Model file for the job. Use its own axes, mm. Face numbers are marked on the shaded views. Coordinates: 2 decimals unless noted, no trailing zeros. Order: outer loops, then holes, each group sorted by start corner. A loop starts at its lowest first (then second) coordinate and runs counter-clockwise, first axis right, second up. Notation, with made-up numbers: M 25,52 L 70,52 A20 cw 70,64 Z; hole C -7,-32.5 d4. An arc over 180 degrees is marked long. Return JSON: item names as keys, results as strings.
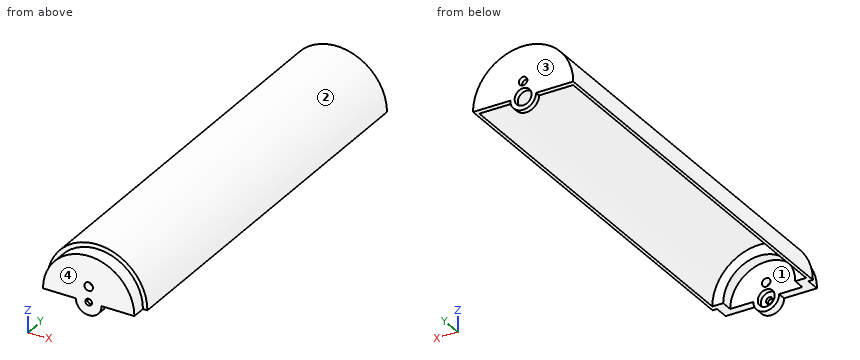
```python
from build123d import *
from build123d.topology import SkipClean

# Parameters (mm, degrees)
BOSS_EXTRUDE1_DEPTH      = 3.81
BOSS_EXTRUDE1_DEPTH_BACK = 6.35
SKETCH1_R                = 49.4538
SKETCH2_R                = 49.4538
BOSS_EXTRUDE2_DEPTH      = 381
SHELL1_T                 = -3.175
CUT_EXTRUDE1_DEPTH       = 398.363186857
BOSS_EXTRUDE3_DEPTH      = 3.81
SKETCH7_R                = 49.4538
SKETCH7_R_2              = 45.085
CUT_EXTRUDE2_DEPTH       = 6.35
BOSS_EXTRUDE4_START      = 7.62
BOSS_EXTRUDE4_DEPTH      = 7.62
SKETCH10_R               = 35.56
CUT_EXTRUDE3_DEPTH       = 6.35
SKETCH11_R               = 8.382
CUT_EXTRUDE4_DEPTH       = 5.08
SKETCH12_R               = 3.302
CUT_EXTRUDE5_DEPTH       = 402.739558289
BOSS_EXTRUDE5_DEPTH      = 5.08
SKETCH14_R               = 4.191
CUT_EXTRUDE6_DEPTH       = 405.866453376
BOSS_EXTRUDE6_DEPTH      = 5.08
SKETCH16_R               = 8.382
CUT_EXTRUDE7_DEPTH       = 405.866453376
CUT_EXTRUDE8_REACH       = 411.871
SKETCH17_R               = 4.191


with BuildPart() as part:
    # Sketch1 → Boss-Extrude1 (new, two sides: drawn at the far end of the back side and taken through both)
    with BuildSketch(Plane(origin=(0, 0, 0), x_dir=(1, 0, 0), z_dir=(0, 1, 0)).offset(-BOSS_EXTRUDE1_DEPTH_BACK)):
        with Locations(Location((0, 0, 0), (0, 0, 270))):
            Circle(SKETCH1_R)
    extrude(amount=BOSS_EXTRUDE1_DEPTH + BOSS_EXTRUDE1_DEPTH_BACK)

    # Sketch2 → Boss-Extrude2 (add)
    with BuildSketch(Plane(origin=(0, 3.81, 0), x_dir=(1, 0, 0), z_dir=(0, 1, 0))):
        with Locations(Location((0, 0, 0), (0, 0, 270))):
            Circle(SKETCH2_R)
    extrude(amount=BOSS_EXTRUDE2_DEPTH)

    # Shell1
    shell1_openings = [part.faces().sort_by_distance(p)[0] for p in [
        (0, 384.81, 0),
    ]]
    offset(amount=SHELL1_T, openings=shell1_openings, kind=Kind.INTERSECTION)

    # Sketch4 → Cut-Extrude1 (cut, through all)
    with BuildSketch(Plane.XZ.offset(6.35)):
        with BuildLine():
            Line((49.4538, 0), (12.7, 0))
            ThreePointArc((12.7, 0), (0, -12.7), (-12.7, 0))
            Line((-12.7, 0), (-49.4538, 0))
            ThreePointArc((-49.4538, 0), (0, -49.4538), (49.4538, 0))
        make_face()
    extrude(amount=-CUT_EXTRUDE1_DEPTH, mode=Mode.SUBTRACT)

    # Sketch5 → Boss-Extrude3 (add)
    with BuildSketch(Plane(origin=(0, -3.175, 0), x_dir=(1, 0, 0), z_dir=(0, 1, 0))):
        with BuildLine():
            Line((-46.2788, 0), (-12.7, 0))
            ThreePointArc((-12.7, 0), (0, 12.7), (12.7, 0))
            Line((12.7, 0), (46.2788, 0))
            ThreePointArc((46.2788, 0), (0, -46.2788), (-46.2788, 0))
        make_face()
    extrude(amount=BOSS_EXTRUDE3_DEPTH)

    # Sketch7 → Cut-Extrude2 (cut)
    with BuildSketch(Plane.XZ.offset(6.35)):
        Circle(SKETCH7_R)
        Circle(SKETCH7_R_2, mode=Mode.SUBTRACT)
    extrude(amount=-CUT_EXTRUDE2_DEPTH, mode=Mode.SUBTRACT)

    # Sketch9 → Boss-Extrude4 (add)
    with SkipClean():  # the faces are left unmerged after this step: merging them gives an invalid solid
        with BuildSketch(Plane.XZ.offset(6.35).offset(BOSS_EXTRUDE4_START)):
            with BuildLine():
                Line((45.085, 0), (12.7, 0))
                ThreePointArc((12.7, 0), (0, -12.7), (-12.7, 0))
                Line((-12.7, 0), (-45.085, 0))
                ThreePointArc((-45.085, 0), (0, 45.085), (45.085, 0))
            make_face()
        extrude(amount=-BOSS_EXTRUDE4_DEPTH)
    add(part.part.scale(1), mode=Mode.REPLACE)  # the faces are merged on a copy

    # Sketch10 → Cut-Extrude3 (cut)
    with BuildSketch(Plane(origin=(0, 0.635, 0), x_dir=(1, 0, 0), z_dir=(0, 1, 0))):
        Circle(SKETCH10_R)
    extrude(amount=-CUT_EXTRUDE3_DEPTH, mode=Mode.SUBTRACT)

    # Sketch11 → Cut-Extrude4 (cut)
    with BuildSketch(Plane(origin=(0, -5.715, 0), x_dir=(1, 0, 0), z_dir=(0, 1, 0))):
        with Locations(Location((0, 0, 0), (0, 0, 270))):
            Circle(SKETCH11_R)
    extrude(amount=-CUT_EXTRUDE4_DEPTH, mode=Mode.SUBTRACT)

    # Sketch12 → Cut-Extrude5 (cut, through all)
    with BuildSketch(Plane(origin=(0, -10.795, 0), x_dir=(1, 0, 0), z_dir=(0, 1, 0))):
        with Locations(Location((0, 0, 0), (0, 0, 270))):
            Circle(SKETCH12_R)
    extrude(amount=-CUT_EXTRUDE5_DEPTH, mode=Mode.SUBTRACT)

    # Sketch13 → Boss-Extrude5 (add)
    with SkipClean():  # the faces are left unmerged after this step: merging them gives an invalid solid
        with BuildSketch(Plane(origin=(0, 0.635, 0), x_dir=(1, 0, 0), z_dir=(0, 1, 0))):
            with BuildLine():
                Line((-46.2788, 0), (-35.56, 0))
                ThreePointArc((-35.56, 0), (0, -35.56), (35.56, 0))
                Line((35.56, 0), (46.2788, 0))
                ThreePointArc((46.2788, 0), (0, -46.2788), (-46.2788, 0))
            make_face()
        extrude(amount=BOSS_EXTRUDE5_DEPTH)
    add(part.part.scale(1), mode=Mode.REPLACE)  # the faces are merged on a copy

    # Sketch14 → Cut-Extrude6 (cut, through all)
    with BuildSketch(Plane.XZ.offset(13.97)):
        with Locations(Location((0, 15.24, 0), (0, 0, 270))):
            Circle(SKETCH14_R)
    extrude(amount=-CUT_EXTRUDE6_DEPTH, mode=Mode.SUBTRACT)

    # Sketch15 → Boss-Extrude6 (add)
    with BuildSketch(Plane(origin=(0, 384.81, 0), x_dir=(1, 0, 0), z_dir=(0, 1, 0))):
        with BuildLine():
            Line((46.2788, 0), (35.56, 0))
            Line((35.56, 0), (12.7, 0))
            ThreePointArc((12.7, 0), (0, 12.7), (-12.7, 0))
            Line((-12.7, 0), (-35.56, 0))
            Line((-35.56, 0), (-46.2788, 0))
            Line((-46.2788, 0), (-49.4538, 0))
            ThreePointArc((-49.4538, 0), (0, -49.4538), (49.4538, 0))
            Line((49.4538, 0), (46.2788, 0))
        make_face()
    extrude(amount=BOSS_EXTRUDE6_DEPTH)

    # Sketch16 → Cut-Extrude7 (cut, through all)
    with BuildSketch(Plane.XZ.offset(-384.81)):
        with Locations(Location((0, 0, 0), (0, 0, 90))):
            Circle(SKETCH16_R)
    extrude(amount=-CUT_EXTRUDE7_DEPTH, mode=Mode.SUBTRACT)

    # Sketch17 → Cut-Extrude8 (cut, up to next)
    with BuildSketch(Plane(origin=(0, 389.89, 0), x_dir=(1, 0, 0), z_dir=(0, 1, 0)), mode=Mode.PRIVATE) as cut_extrude8_sk1:
        with Locations(Location((0, -15.24, 0), (0, 0, 90))):
            Circle(SKETCH17_R)
    cut_extrude8_tool1 = extrude(cut_extrude8_sk1.sketch, amount=-CUT_EXTRUDE8_REACH, mode=Mode.PRIVATE) & part.part
    add(cut_extrude8_tool1.solids().sort_by_distance((0, 389.89, 15.24))[0], mode=Mode.SUBTRACT)


solid = part.part
```
Item 1: Saw through at D-D (x = 39.5). Write the cut outline in (y, z) (3 decimals), and give its area (3 significant figures).
Check result:
{"outline": "M -13.97,0 L 5.715,0 L 5.715,24.114 L 384.81,24.114 L 384.81,0 L 389.89,0 L 389.89,29.756 L 0,29.756 L 0,21.735 L -13.97,21.735 Z", "area": "2,760 mm2"}
Item 2: Saw through at A-A (z = 15.24). Write the cut outline in (x, y) (3 decimals).
Check result:
{"outline": "M -47.047,0 L -42.431,0 L -42.431,-13.97 L -4.191,-13.97 L -4.191,-5.715 L -32.129,-5.715 L -32.129,5.715 L -43.697,5.715 L -43.697,384.81 L -4.191,384.81 L -4.191,389.89 L -47.047,389.89 Z; M 4.191,-13.97 L 42.431,-13.97 L 42.431,0 L 47.047,0 L 47.047,389.89 L 4.191,389.89 L 4.191,384.81 L 43.697,384.81 L 43.697,5.715 L 32.129,5.715 L 32.129,-5.715 L 4.191,-5.715 Z"}
Item 3: Wall check: line 1 (Y direction, x = 5, z = 40) (3 decimals); line 2 (X direction, y = 7, z = 2.5); line 3 (Z direction, x = 0, y = 334.5). Give the ranges that are in metal, low to high.
Check result:
{"line 1": "y = -13.97 to 5.715, 384.81 to 389.89", "line 2": "x = -49.39 to -46.21, 46.21 to 49.39", "line 3": "z = 46.28 to 49.45"}
Item 4: Drop flat-ended pins along their axis: pin 1 Ø10 at (y, z) = (151, 10.5) entering from +X; pin 2 Ø5 at (x, y) = (17.5, 226.5) entering from -Z; pin 3 Ø1 at (y, z) = (254, 34) entering from +X; pin 4 Ø13.5 at (x, z) = (0, 15.24) entering from -Y. Give the stop position or say it passes through.
Check result:
{"pin 1": "stops at x = 49.15", "pin 2": "stops at z = 41.73", "pin 3": "stops at x = 36.38", "pin 4": "stops at y = -13.97"}
Item 5: Saw through at B-B (x = -28.5). Write the cut outline in (y, z) (1 decimal), and give its area (3 significant figures).
Check result:
{"outline": "M -14,0 L -5.7,0 L -5.7,21.3 L 5.7,21.3 L 5.7,36.5 L 384.8,36.5 L 384.8,0 L 389.9,0 L 389.9,40.4 L 0,40.4 L 0,34.9 L -14,34.9 Z", "area": "2,180 mm2"}
Item 6: Pull direction Y, two halves, no side cores. Call the marked faces 1, 2, 3 and 4: +Y half, -Y half, draft (parallel to the pull), parting line (faces both ways), or undercut.
Check result:
{"face 1": "undercut", "face 2": "draft", "face 3": "+Y half", "face 4": "-Y half"}
Item 7: Saw through at C-C (y = 55). Write the cut outline in (x, z), and give its area (3 significant figures).
Check result:
{"outline": "M -49.45,0 L -46.28,0 A46.28 cw 46.28,0 L 49.45,0 A49.45 ccw Z", "area": "477 mm2"}
